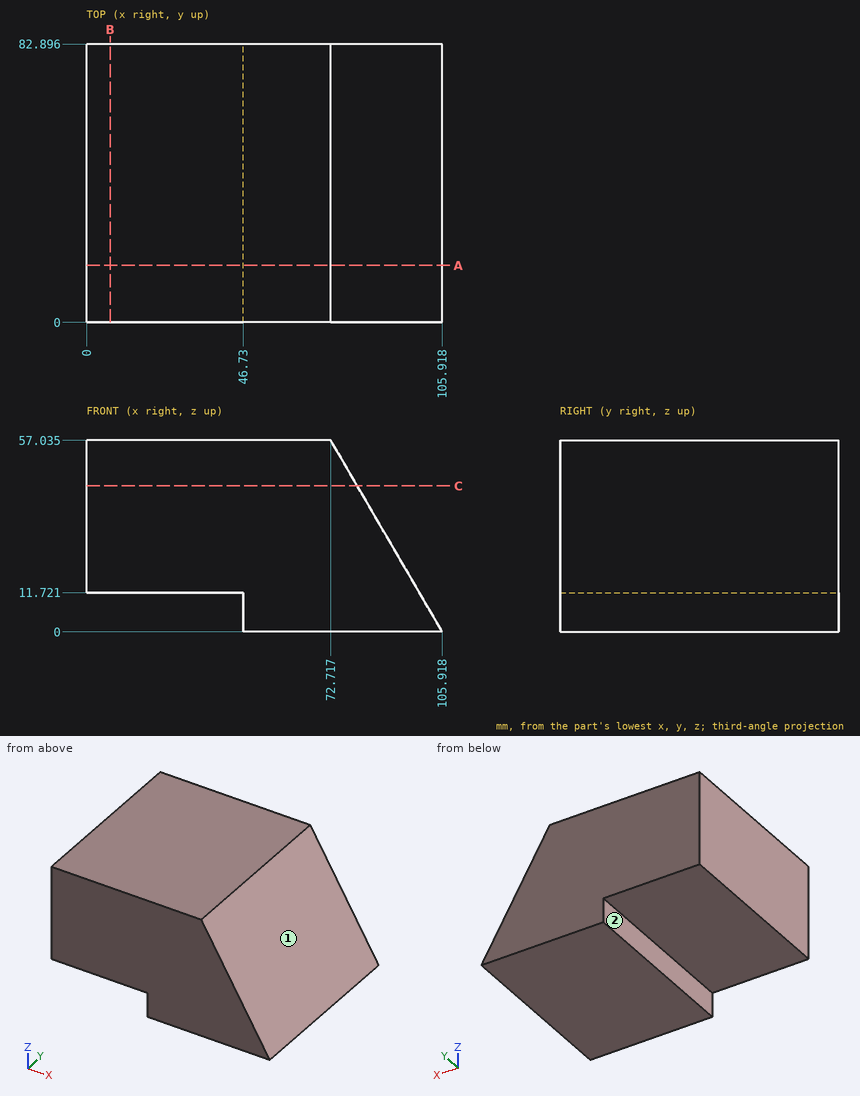
Geometry: see drawing. Coordinates: mm, zero at the bounding-box minimum. A direction names the side the tool comes from. Coordinates: 2 decimals unless noted, no trailing zeros. Order: outer loops, then holes, each group sorted by start corner. A loop starts at its lowest first (then second) coordinate and runs counter-clockwise, first axis right, second up. Notation, with made-up numbers: (4, 16.25) - (54, 16.25) arc R34 ccw to (54, 46.25) - close; hole circle Ø4 at (79, 40.25). An arc over 180 degrees is marked (long way). Use one line per item in the form item = value.
1) Pin query (flat end, axial travel): pin 1 (1 mm diameter, centred on y = 35.5, z = 49, fed in from +X) (1 decimal); pin 2 (10 mm diameter, centred on y = 64.5, z = 48, fed in from +X); pin 3 (6 mm diameter, centred on y = 11, z = 23.5, fed in from +X) (1 decimal). Return the tip coordinate at first contact, or that it passes through.
Solutions:
pin_1 = 77.7
pin_2 = 80.89
pin_3 = 94
2) Set-up query: the marked faces 1 and 2. Return all of +Z, -Z, +X, -X, +Y, -Y with unobstructed straight access to the full face (end or side cutting, diameter ignored); none if empty.
Solutions:
face_1 = +Z, +X, +Y, -Y
face_2 = -Z, -X, +Y, -Y
3) Ray query, L1, parallel to Z at x = 27.5, y = 41.5 (1 decimal); L2, parallel to Z at x = 79, y = 42 (1 decimal); L3, parallel to X at y = 28.5, z = 22.5. Return the intervals inside material, ascending.
Solutions:
L1 = 11.7 to 57
L2 = 0 to 46.2
L3 = 0 to 92.82
4) Section A-A (y = 17). Return loops of the section in (x, z) (1 decimal).
Solutions:
outline = (0, 11.7) - (46.7, 11.7) - (46.7, 0) - (105.9, 0) - (72.7, 57) - (0, 57) - close
5) Section B-B (x = 7). Return loops of the section in (y, z) (1 decimal), then the cut area to 3 significant figures.
Solutions:
outline = (0, 11.7) - (82.9, 11.7) - (82.9, 57) - (0, 57) - close
area = 3,760 mm^2
6) Section C-C (z = 43.5). Return loops of the section in (x, y).
Solutions:
outline = (0, 0) - (80.6, 0) - (80.6, 82.9) - (0, 82.9) - close
